from build123d import *

# Parameters (mm, degrees)
SKETCH1_W          = 70
SKETCH1_H          = 1.2
SKETCH4_W          = 70
SKETCH4_H          = 1.2
CUT_EXTRUDE3_DEPTH = 900


with BuildPart() as part:
    # Sweep1: sweep along a path in Sketch2
    with BuildLine(Plane(origin=(0, 0, 0), x_dir=(-1, 0, 0), z_dir=(0, 1, 0))) as sweep1_path:
        Line((0, 0), (999.171572875, 0))
        ThreePointArc((999.171572875, 0), (999.93693974, -0.152240935), (1000.585786438, -0.585786438))
        Line((1000.585786438, -0.585786438), (1006.290281407, -6.290281407))
        ThreePointArc((1006.290281407, -6.290281407), (1006.939128104, -6.723826909), (1007.704494969, -6.876067844))
        Line((1007.704494969, -6.876067844), (1080.606989687, -6.876067844))
        ThreePointArc((1080.606989687, -6.876067844), (1082.706989687, -4.776067844), (1080.606989687, -2.676067844))
        Line((1080.606989687, -2.676067844), (1008.876067844, -2.676067844))
        ThreePointArc((1008.876067844, -2.676067844), (1007.461854282, -2.090281407), (1006.876067844, -0.676067844))
        Line((1006.876067844, -0.676067844), (1006.876067844, 16.495505031))
        ThreePointArc((1006.876067844, 16.495505031), (1006.723826909, 17.260871896), (1006.290281407, 17.909718593))
        Line((1006.290281407, 17.909718593), (993.319718658, 30.880281342))
        ThreePointArc((993.319718658, 30.880281342), (992.886173156, 31.529128039), (992.733932221, 32.294494904))
        Line((992.733932221, 32.294494904), (992.733932221, 49.466067779))
        ThreePointArc((992.733932221, 49.466067779), (992.148145783, 50.880281342), (990.733932221, 51.466067779))
        Line((990.733932221, 51.466067779), (972.733932221, 51.466067779))
    # Sketch1 → Sweep1 (sweep)
    with BuildSketch(Plane.YZ):
        Rectangle(SKETCH1_W, SKETCH1_H)
    sweep(path=sweep1_path.line)

    # Sketch4 → Cut-Extrude3 (cut)
    with BuildSketch(Plane.YZ):
        Rectangle(SKETCH4_W, SKETCH4_H)
    extrude(amount=-CUT_EXTRUDE3_DEPTH, mode=Mode.SUBTRACT)


solid = part.part
Design review of the part built by this model. Coordinates are the model's own, in mm. A direction names the side the tool comes from. Round coordinates to 2 decimals unless told otherwise and drop trailing zeros. Order: outer loops, then holes, each group sorted by start corner. A loop starts at its lowest first (then second) coordinate and runs counter-clockwise, first axis right, second up. Notation, with made-up numbers: M 27.5,63 L 44.5,63 A11 ccw 44.5,73 Z; hole C 78,7 d2. An arc over 180 degrees is marked long. Answer as CSV lines item,"result". Start each with the question number.
1) Add section D-D (z = 44). Give the boundary of the cut face in (x, y), then the cut area to 3 significant figures.
2) The part is to be moulded in two halves that separate along Z. For faces 5 (the face through (-950, 0, 0.6)), 6 (the face through (-993.334, 0, 41)), 7 (the face through (-950, 0, -0.6)), say which applies: +Z half, -Z half, draft (parallel to the pull), parting line (faces both ways), or undercut.
3) Tool access review of faces 1 (the face through (-1045, 0, -6.276)), 2 (the face through (-1083.306, 0.49, -4.835)), 3 (the face through (-1044, 0, -2.076)), 4 (the face through (-999.29, 0.49, 24.06)): name each direction out of +Z, -Z, +X, -X, +Y, -Y from which nothing blocks a thin tool from reaching the whole face with its end or side.
4) Add section C-C (x = -995.5). Give the boundary of the cut face in (y, z).
5) Wall thickness on line 1 along Z through (x, y) = (-1033, -13); line 2 along X through (y, z) = (-23, 7.5); line 3 along X through (y, z) = (16, 46): over which ranges is each line inside the solid? List them lowest first. Write a range as [from, to].
6) Add section A-A (x = -1051). Give the boundary of the cut face in (y, z).
7) For pin 1 Ø5 at (y, z) = (-21, 19) entering from -X; pin 2 Ø8 at (y, z) = (-25.5, 16.5) entering from +X; pin 3 Ø12 at (y, z) = (23.5, 40) entering from +X, all flat-tipped, find the tip position at first contact; note any pin that passes through.
Resolved:
1,outline,"M -993.33,-35 L -992.13,-35 L -992.13,35 L -993.33,35 Z"
1,area,"84.0 mm^2"
2,face 5,"undercut"
2,face 6,"draft"
2,face 7,"-Z half"
3,face 1,"+Y, -Y"
3,face 2,"-X, +Y, -Y"
3,face 3,"+Z, -X, +Y, -Y"
3,face 4,"+X, +Y, -Y"
4,outline,"M -35,-0.6 L 35,-0.6 L 35,0.6 L -35,0.6 Z; M -35,27.85 L 35,27.85 L 35,29.55 L -35,29.55 Z"
5,line 1,"[-7.48, -6.28], [-3.28, -2.08]"
5,line 2,"[-1007.48, -1006.28]"
5,line 3,"[-993.33, -992.13]"
6,outline,"M -35,-7.48 L 35,-7.48 L 35,-6.28 L -35,-6.28 Z; M -35,-3.28 L 35,-3.28 L 35,-2.08 L -35,-2.08 Z"
7,pin 1,"x = -1007.48"
7,pin 2,"x = -1002.85"
7,pin 3,"x = -992.13"
